Geometry check sheet. Reference: the model listing, model coordinates, mm. Coordinates: 2 decimals unless noted, no trailing zeros. Loops run counter-clockwise (first coordinate to the right, second up) from the corner with the lowest first, then second, coordinate; pieces in that order, holes last. Notation, with made-up numbers: (86.25, 60.5) -> (128.25, 60.5) arc R6 ccw to (128.25, 65.5) -> close; hole circle Ø9 at (65.25, -5.5). An arc over 180 degrees is marked (long way). Answer as a JSON object with one key per item and string values.
from build123d import *

# Parameters (mm, degrees)
SKETCH_1_R          = 1.6
SKETCH_1_W          = 45.5
SKETCH_1_H          = 2.2
SKETCH_1_W_2        = 2.2
SKETCH_1_H_2        = 50.5
SKETCH_1_W_3        = 12.2
SKETCH_1_R_2        = 7.08
EXTRUDE_1_DEPTH     = 2
SKETCH_2_W          = 4
SKETCH_2_H          = 160
CUT_EXTRUDE_1_DEPTH = 10
SKETCH_3_R          = 1.6
CUT_EXTRUDE_2_DEPTH = 10
FILLET_1_R          = 3


with BuildPart() as part:
    # 草图1 → 凸台-拉伸1 (new body)
    with BuildSketch(Plane.XY):
        with BuildLine():
            Line((-8.65326359, -109.246690295), (-8.65326359, -85.5))
            Line((-8.65326359, -85.5), (11, -85.5))
            Line((11, -85.5), (11, 74.5))
            Line((11, 74.5), (-11, 74.5))
            Line((-11, 74.5), (-11, -74.5))
            Line((-11, -74.5), (-59, -74.5))
            Line((-59, -74.5), (-59, -80.5))
            Line((-59, -80.5), (-45.65326359, -80.5))
            Line((-45.65326359, -80.5), (-45.65326359, -109.246690295))
            ThreePointArc((-45.65326359, -109.246690295), (-42.686252119, -119.728927736), (-34.665533413, -127.101073304))
            Line((-34.665533413, -127.101073304), (-34.351105887, -127.259785353))
            ThreePointArc((-34.351105887, -127.259785353), (-27.15326359, -128.973428312), (-19.955421292, -127.259785353))
            Line((-19.955421292, -127.259785353), (-19.640993767, -127.101073304))
            ThreePointArc((-19.640993767, -127.101073304), (-11.620275061, -119.728927736), (-8.65326359, -109.246690295))
        make_face()
        with Locations((-11, -81.629391896)):
            Circle(SKETCH_1_R, mode=Mode.SUBTRACT)
        with Locations((-42.570682945, -81.629391896)):
            Circle(SKETCH_1_R, mode=Mode.SUBTRACT)
        with Locations((-42.65326359, -106)):
            Circle(SKETCH_1_R, mode=Mode.SUBTRACT)
        with Locations((-34.90326359, -92.576606241)):
            Circle(SKETCH_1_R, mode=Mode.SUBTRACT)
        with Locations((-19.40326359, -92.576606241)):
            Circle(SKETCH_1_R, mode=Mode.SUBTRACT)
        with Locations((-11.65326359, -106)):
            Circle(SKETCH_1_R, mode=Mode.SUBTRACT)
        with Locations((-19.40326359, -119.423393759)):
            Circle(SKETCH_1_R, mode=Mode.SUBTRACT)
        with Locations((-34.90326359, -119.423393759)):
            Circle(SKETCH_1_R, mode=Mode.SUBTRACT)
        with Locations((-21.75, -77.5)):
            Rectangle(SKETCH_1_W, SKETCH_1_H, mode=Mode.SUBTRACT)
        with Locations((3.8, 61.7)):
            Circle(SKETCH_1_R, mode=Mode.SUBTRACT)
        with Locations((-4, -71.5)):
            Circle(SKETCH_1_R, mode=Mode.SUBTRACT)
        with Locations((3.8, -71.5)):
            Circle(SKETCH_1_R, mode=Mode.SUBTRACT)
        with Locations((-4, -51.5)):
            Circle(SKETCH_1_R, mode=Mode.SUBTRACT)
        with Locations((3.8, -51.5)):
            Circle(SKETCH_1_R, mode=Mode.SUBTRACT)
        with Locations((0, -17.25)):
            Rectangle(SKETCH_1_W_2, SKETCH_1_H_2, mode=Mode.SUBTRACT)
        with Locations((-4, -0.5)):
            Circle(SKETCH_1_R, mode=Mode.SUBTRACT)
        with Locations((3.8, -0.5)):
            Circle(SKETCH_1_R, mode=Mode.SUBTRACT)
        with Locations((-4, 61.7)):
            Circle(SKETCH_1_R, mode=Mode.SUBTRACT)
        with Locations((-0.1, 66.4)):
            Rectangle(SKETCH_1_W_3, SKETCH_1_H, mode=Mode.SUBTRACT)
        with Locations((-27.15326359, -113)):
            Circle(SKETCH_1_R_2, mode=Mode.SUBTRACT)
    extrude(amount=EXTRUDE_1_DEPTH)

    # 草图2 → 切除-拉伸1 (cut)
    with BuildSketch(Plane(origin=(0, 0, 0), x_dir=(-1, 0, 0), z_dir=(0, 0, -1))):
        with Locations((-9, -5.5)):
            Rectangle(SKETCH_2_W, SKETCH_2_H)
    extrude(amount=-CUT_EXTRUDE_1_DEPTH, mode=Mode.SUBTRACT)

    # 草图3 → 切除-拉伸2 (cut)
    with BuildSketch(Plane(origin=(0, 0, 0), x_dir=(-1, 0, 0), z_dir=(0, 0, -1))):
        with Locations((-4, -82.5)):
            Circle(SKETCH_3_R)
    extrude(amount=-CUT_EXTRUDE_2_DEPTH, mode=Mode.SUBTRACT)

    # 圆角1
    fillet_1_edges = [part.edges().sort_by_distance(p)[0] for p in [
        (7, 74.5, 1),
        (-11, 74.5, 1),
        (-59, -74.5, 1),
        (-59, -80.5, 1),
        (7, -85.5, 1),
    ]]
    fillet(fillet_1_edges, radius=FILLET_1_R - 0.0001)  # a hair under: the kernel refuses the full size


solid = part.part
1. Section check D-D, the plane z = 0.7. State how many separate pieces and enclosed holes the cut face has, then the cut area to 3 significant figures.
Evaluation:
{"separate pieces": "1", "enclosed holes": "21", "area": "4,250 mm^2"}
2. Section check A-A, the plane y = -17. Record the boundary of the cut face in (x, z).
Evaluation:
{"outline": "(-11, 0) -> (-1.1, 0) -> (-1.1, 2) -> (-11, 2) -> close; (1.1, 0) -> (7, 0) -> (7, 2) -> (1.1, 2) -> close"}
3. Section check C-C, the plane y = -68. Record the boundary of the cut face in (x, z), then the cut area to 3 significant figures.
Evaluation:
{"outline": "(-11, 0) -> (7, 0) -> (7, 2) -> (-11, 2) -> close", "area": "36.0 mm^2"}
4. Depth check by flat-ended pin: P1, Ø6, axis at x = -11, y = -70.5, coming from the -Z side; P2, Ø1, axis at x = -42, z = 1, coming from the +Y side; P3, Ø1, axis at x = -1, z = 1.5, coming from the -Y side; P4, Ø1, axis at y = -96.5, z = 1, coming from the -X side. Enter the tip coordinate at first touch or a pass-through.
Evaluation:
{"P1": "stops at z = 0", "P2": "stops at y = -74.5", "P3": "stops at y = -85.5", "P4": "stops at x = -45.65"}
5. Section check B-B, the plane x = -30. Record the boundary of the cut face in (y, z).
Evaluation:
{"outline": "(-128.72, 0) -> (-119.48, 0) -> (-119.48, 2) -> (-128.72, 2) -> close; (-106.52, 0) -> (-78.6, 0) -> (-78.6, 2) -> (-106.52, 2) -> close; (-76.4, 0) -> (-74.5, 0) -> (-74.5, 2) -> (-76.4, 2) -> close"}
6. Mould release check, pull along X, two halves, no side actions. Record for faces 1 (the face through (-42.767, -119.597, 0.986)), 2 (the face through (-7, -34, 0)), 3 (the face through (-32.77, -117.31, 0.99)): released by +X, released by -X, zero draft, split by the parting line, or undercut.
Evaluation:
{"face 1": "released by -X", "face 2": "zero draft", "face 3": "undercut"}
7. Thickness scan on probe 1 along Y at (x, z) = (-27, 1.65); probe 2 along Y at (x, z) = (-28, 1.3); probe 3 along X at (y, z) = (-29, 1.3). Record the ranges inside material, lowest first. Write a range as from..to.
Evaluation:
{"probe 1": "y = -128.97..-120.08, -105.92..-78.6, -76.4..-74.5", "probe 2": "y = -128.95..-120.03, -105.97..-78.6, -76.4..-74.5", "probe 3": "x = -11..-1.1, 1.1..7"}
